```python
from build123d import *
from build123d.topology import SkipClean

# Parameters (mm, degrees)
BOSS_EXTRUDE1_DEPTH  = 10
CHAMFER1_SIZE        = 3
M4_CLEARANCE_HOLE1_D = 4.8
CUT_EXTRUDE1_START   = -8
SKETCH4_R            = 3.7
SKETCH4_R_2          = 2.4
CUT_EXTRUDE1_DEPTH   = 8
SKETCH4_3_R          = 3.7
SKETCH4_3_R_2        = 2.4
CUT_EXTRUDE2_DEPTH   = 28.935018749
CUT_EXTRUDE3_DEPTH   = 3


with BuildPart() as part:
    # Sketch1 → Boss-Extrude1 (new body)
    with BuildSketch(Plane(origin=(0, 0, 0), x_dir=(1, 0, 0), z_dir=(0, 1, 0))):
        with BuildLine():
            ThreePointArc((4.929173178, -18.444040543), (0, -15.55551692), (-4.929173178, -18.444040543))
            ThreePointArc((-4.929173178, -18.444040543), (-7.30594069, -17.6381011), (-9.556454361, -16.527357921))
            ThreePointArc((-9.556454361, -16.527357921), (-10.999411499, -10.999411499), (-16.527357921, -9.556454361))
            ThreePointArc((-16.527357921, -9.556454361), (-17.6381011, -7.30594069), (-18.444040543, -4.929173178))
            ThreePointArc((-18.444040543, -4.929173178), (-15.55551692, 0), (-18.444040543, 4.929173178))
            ThreePointArc((-18.444040543, 4.929173178), (-17.6381011, 7.30594069), (-16.527357921, 9.556454361))
            ThreePointArc((-16.527357921, 9.556454361), (-10.999411499, 10.999411499), (-9.556454361, 16.527357921))
            ThreePointArc((-9.556454361, 16.527357921), (-7.30594069, 17.6381011), (-4.929173178, 18.444040543))
            ThreePointArc((-4.929173178, 18.444040543), (0, 15.55551692), (4.929173178, 18.444040543))
            ThreePointArc((4.929173178, 18.444040543), (7.30594069, 17.6381011), (9.556454361, 16.527357921))
            ThreePointArc((9.556454361, 16.527357921), (10.999411499, 10.999411499), (16.527357921, 9.556454361))
            ThreePointArc((16.527357921, 9.556454361), (17.6381011, 7.30594069), (18.444040543, 4.929173178))
            ThreePointArc((18.444040543, 4.929173178), (15.55551692, 0), (18.444040543, -4.929173178))
            ThreePointArc((18.444040543, -4.929173178), (17.6381011, -7.30594069), (16.527357921, -9.556454361))
            ThreePointArc((16.527357921, -9.556454361), (10.999411499, -10.999411499), (9.556454361, -16.527357921))
            ThreePointArc((9.556454361, -16.527357921), (7.30594069, -17.6381011), (4.929173178, -18.444040543))
        make_face()
    extrude(amount=BOSS_EXTRUDE1_DEPTH)

    # Chamfer1
    chamfer1_edges = [part.edges().sort_by_distance(p)[0] for p in [
        (7.30594069, 10, -17.6381011),
        (17.6381011, 0, 7.30594069),
        (7.30594069, 0, 17.6381011),
        (-7.30594069, 0, 17.6381011),
        (-17.6381011, 0, 7.30594069),
        (-17.6381011, 0, -7.30594069),
        (-7.30594069, 0, -17.6381011),
        (-7.30594069, 10, -17.6381011),
        (7.30594069, 0, -17.6381011),
        (17.6381011, 0, -7.30594069),
        (-17.6381011, 10, -7.30594069),
        (-17.6381011, 10, 7.30594069),
        (-7.30594069, 10, 17.6381011),
        (17.6381011, 10, -7.30594069),
        (7.30594069, 10, 17.6381011),
        (17.6381011, 10, 7.30594069),
    ]]
    chamfer(chamfer1_edges, length=CHAMFER1_SIZE)

    # M4 Clearance Hole1 (through all)
    with Locations(Plane(origin=(0, 10, 0), x_dir=(1, 0, 0), z_dir=(0, 1, 0))):
        with Locations((0, 0)):
            Hole(M4_CLEARANCE_HOLE1_D / 2)

    # Sketch4 → Cut-Extrude1 (cut)
    # profile 1 of 4: a face of its own
    with BuildSketch(Plane(origin=(0, 10, 0), x_dir=(1, 0, 0), z_dir=(0, 1, 0)).offset(CUT_EXTRUDE1_START)):
        with BuildLine():
            ThreePointArc((-11.865806229, 7.290510339), (-14.597296614, 6.046398231), (-13.545561348, 3.23522275))
            Line((-13.545561348, 3.23522275), (-3.148841491, -1.94288375))
            ThreePointArc((-3.148841491, -1.94288375), (-3.41835427, 1.4159287), (-0.852740897, 3.600393446))
            Line((-0.852740897, 3.600393446), (-11.865806229, 7.290510339))
        make_face()
    # profile 2 of 4: a face of its own
    with BuildSketch(Plane(origin=(0, 10, 0), x_dir=(1, 0, 0), z_dir=(0, 1, 0)).offset(CUT_EXTRUDE1_START)):
        Circle(SKETCH4_R)
        with Locations(Location((0, 0, 0), (0, 0, 270))):
            Circle(SKETCH4_R_2, mode=Mode.SUBTRACT)
    # profile 3 of 4: a face of its own
    with BuildSketch(Plane(origin=(0, 10, 0), x_dir=(1, 0, 0), z_dir=(0, 1, 0)).offset(CUT_EXTRUDE1_START)):
        with Locations(Location((0, 0, 0), (0, 0, 270))):
            Circle(SKETCH4_R_2)
    # profile 4 of 4: a face of its own
    with BuildSketch(Plane(origin=(0, 10, 0), x_dir=(1, 0, 0), z_dir=(0, 1, 0)).offset(CUT_EXTRUDE1_START)):
        with BuildLine():
            ThreePointArc((3.7, 0), (2.902166546, -2.29508809), (0.852740897, -3.600393446))
            Line((0.852740897, -3.600393446), (11.865806229, -7.290510339))
            ThreePointArc((11.865806229, -7.290510339), (14.597296614, -6.046398231), (13.545561348, -3.23522275))
            Line((13.545561348, -3.23522275), (3.148841491, 1.94288375))
            ThreePointArc((3.148841491, 1.94288375), (3.559544459, 1.009773857), (3.7, 0))
        make_face()
    extrude(amount=CUT_EXTRUDE1_DEPTH, mode=Mode.SUBTRACT)

    # Sketch4<3> → Cut-Extrude2 (cut, through all)
    # profile 1 of 2: a face of its own
    with SkipClean():  # the faces are left unmerged after this step: merging them gives an invalid solid
        with BuildSketch(Plane(origin=(0, 10, 0), x_dir=(1, 0, 0), z_dir=(0, 1, 0))):
            with Locations(Location((0, 0, 0), (0, 0, 270))):
                Circle(SKETCH4_3_R)
            Circle(SKETCH4_3_R_2, mode=Mode.SUBTRACT)
        # profile 2 of 2: a face of its own
        with BuildSketch(Plane(origin=(0, 10, 0), x_dir=(1, 0, 0), z_dir=(0, 1, 0))):
            Circle(SKETCH4_3_R_2)
        extrude(amount=-CUT_EXTRUDE2_DEPTH, mode=Mode.SUBTRACT)

    # Sketch5 → Cut-Extrude3 (cut)
    with SkipClean():  # the faces are left unmerged after this step: merging them gives an invalid solid
        with BuildSketch(Plane(origin=(0, 10, 0), x_dir=(1, 0, 0), z_dir=(0, 1, 0))):
            Polygon((2.165063509, -3.75), (4.330127019, 0), (2.165063509, 3.75), (-2.165063509, 3.75), (-4.330127019, 0), (-2.165063509, -3.75), align=None)
        extrude(amount=-CUT_EXTRUDE3_DEPTH, mode=Mode.SUBTRACT)


solid = part.part
```
The listing builds one solid part. Answer for the finished solid, in the listing's coordinates (mm). A direction names the side the tool comes from. Coordinates: 2 decimals unless noted, no trailing zeros. Loops run counter-clockwise (first coordinate to the right, second up) from the corner with the lowest first, then second, coordinate; pieces in that order, holes last. Notation, with made-up numbers: (69, 75.5) -> (91, 75.5) arc R22 cw to (91, 103.5) -> close; hole circle Ø11 at (-17.75, 15.25). An arc over 180 degrees is marked (long way). Return JSON: item names as keys, results as strings. Group by question number.
(1) Which of the six approach directions +Z, -Z, +X, -X, +Y, -Y give full straight-line access (tool end or side, diameter ignored) to faces 1 (the flat face through (8.42, 5.944, 0.682)), 2 (the cylindrical face through (11, 5, 11))?
(2) A cutting plane is placed at A-A on y = 5. Write down the section's boundary in (x, z), and give its area (3 significant figures).
(3) Given pin 1 Ø2.5 at (x, y) = (-1, 8) entering from -Z; pin 2 Ø1 at (y, z) = (1.5, -13.5) entering from -X; pin 3 Ø1.5 at (y, z) = (5.5, 6) entering from +X, each flat-ended and moving along its own axis, determine where each tip first touches the part or whether it passes through.
(4) Find the intervals of material crossed by probe 1 along Z at (x, y) = (-2.5, 5.5); probe 2 along Z at (x, y) = (-16, 4.75); probe 3 along X at (y, z) = (6.5, 2), in increasing order. Write a range as from..to.
(5) Determine the mould class of faces 3 (the cylindrical face through (-14.58, 5.94, -6.09)), 4 (the cylindrical face through (-7.273, 4.972, 17.652)), 5 (the conical face through (6.54, 8.85, -15.95)) for opening direction Z: released by +Z, released by -Z, zero draft, split by the parting line, or undercut.
(6) A cutting plane is placed at B-B on z = 0. Write down the section's boundary in (x, y).
(7) A cutting plane is placed at C-C on y = 8. Write down the section's boundary in (x, z), and give its area (3 significant figures).
The answers:
{
 "1": {"face 1": "+Y", "face 2": "+Y, -Y"},
 "2": {"outline": "(-18.44, -4.93) arc R19.09 ccw to (-16.53, -9.56) arc R5.65 cw to (-9.56, -16.53) arc R19.09 ccw to (-4.93, -18.44) arc R5.65 cw to (4.93, -18.44) arc R19.09 ccw to (9.56, -16.53) arc R5.65 cw to (16.53, -9.56) arc R19.09 ccw to (18.44, -4.93) arc R5.65 cw to (18.44, 4.93) arc R19.09 ccw to (16.53, 9.56) arc R5.65 cw to (9.56, 16.53) arc R19.09 ccw to (4.93, 18.44) arc R5.65 cw to (-4.93, 18.44) arc R19.09 ccw to (-9.56, 16.53) arc R5.65 cw to (-16.53, 9.56) arc R19.09 ccw to (-18.44, 4.93) arc R5.65 cw to start; hole (-13.55, -3.24) arc R2.2 ccw to (-11.87, -7.29) -> (-0.85, -3.6) arc R3.7 ccw to (3.15, -1.94) -> (13.55, 3.24) arc R2.2 ccw to (11.87, 7.29) -> (0.85, 3.6) arc R3.7 ccw to (-3.15, 1.94) -> close", "area": "785 mm^2"},
 "3": {"pin 1": "stops at z = -16.02", "pin 2": "stops at x = -9.71", "pin 3": "stops at x = 18.36"},
 "4": {"probe 1": "z = -16.14..-4.15, 2.73..16.14", "probe 2": "z = -9.43..-2.2, 2.2..9.43", "probe 3": "x = -15.92..-3.11, 11.07..15.92"},
 "5": {"face 3": "undercut", "face 4": "released by +Z", "face 5": "released by -Z"},
 "6": {"outline": "(-15.56, 0) -> (-3.7, 0) -> (-3.7, 2) -> (-7.05, 2) -> (-7.05, 10) -> (-15.56, 10) -> close; (3.7, 0) -> (15.56, 0) -> (15.56, 10) -> (7.05, 10) -> (7.05, 2) -> (3.7, 2) -> close"},
 "7": {"outline": "(-17.57, -4.32) arc R18.09 ccw to (-15.48, -9.37) arc R5.65 cw to (-9.37, -15.48) arc R18.09 ccw to (-4.32, -17.57) arc R5.65 cw to (4.32, -17.57) arc R18.09 ccw to (9.37, -15.48) arc R5.65 cw to (15.48, -9.37) arc R18.09 ccw to (17.57, -4.32) arc R5.65 cw to (17.57, 4.32) arc R18.09 ccw to (15.48, 9.37) arc R5.65 cw to (9.37, 15.48) arc R18.09 ccw to (4.32, 17.57) arc R5.65 cw to (-4.32, 17.57) arc R18.09 ccw to (-9.37, 15.48) arc R5.65 cw to (-15.48, 9.37) arc R18.09 ccw to (-17.57, 4.32) arc R5.65 cw to start; hole (-13.55, -3.24) arc R2.2 ccw to (-11.87, -7.29) -> (-1.3, -3.75) -> (2.17, -3.75) -> (3.23, -1.9) -> (13.55, 3.24) arc R2.2 ccw to (11.87, 7.29) -> (1.3, 3.75) -> (-2.17, 3.75) -> (-3.23, 1.9) -> close", "area": "741 mm^2"}
}
